```python
from build123d import *

# Parameters (mm, degrees)
PAD_DEPTH    = 4
PAD001_DEPTH = 5
POCKET_DEPTH = 4


with BuildPart() as part:
    # Sketch → Pad (new body)
    with BuildSketch(Plane.XY):
        with BuildLine():
            Line((-7, -50), (7, -50))
            Line((7, -50), (7, 0))
            Line((7, 0), (15, 0))
            ThreePointArc((15, 0), (30, 15), (15, 30))
            Line((15, 30), (-15, 30))
            ThreePointArc((-15, 30), (-30, 15), (-15, 0))
            Line((-15, 0), (-7, 0))
            Line((-7, 0), (-7, -50))
        make_face()
    extrude(amount=PAD_DEPTH)

    # Sketch001 → Pad001 (join)
    with BuildSketch(Plane.XY):
        with BuildLine():
            Line((-6, -50), (6, -50))
            Line((6, -50), (6, 1))
            Line((6, 1), (15, 1))
            ThreePointArc((15, 1), (29, 15), (15, 29))
            Line((15, 29), (-15, 29))
            ThreePointArc((-15, 29), (-29, 15), (-15, 1))
            Line((-15, 1), (-6, 1))
            Line((-6, 1), (-6, -50))
        make_face()
    extrude(amount=PAD001_DEPTH)

    # Sketch002 → Pocket (cut)
    with BuildSketch(Plane.XY.offset(5)):
        with BuildLine():
            Line((-5, -50), (5, -50))
            Line((5, -50), (5, 2))
            Line((5, 2), (15, 2))
            ThreePointArc((15, 2), (28, 15), (15, 28))
            Line((15, 28), (-15, 28))
            ThreePointArc((-15, 28), (-28, 15), (-15, 2))
            Line((-15, 2), (-5, 2))
            Line((-5, 2), (-5, -50))
        make_face()
    extrude(amount=-POCKET_DEPTH, mode=Mode.SUBTRACT)


solid = part.part
```
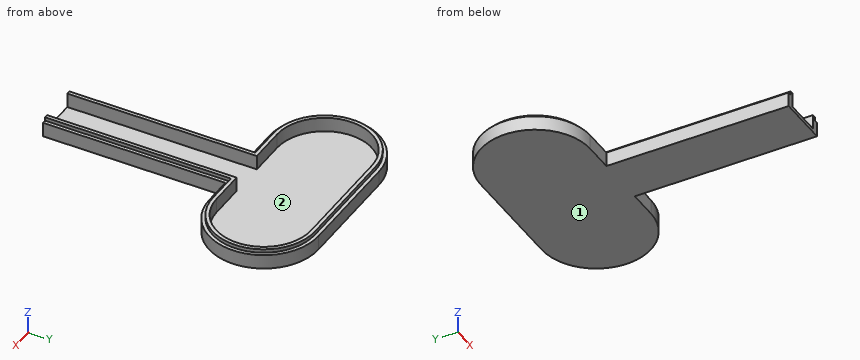
Verification items for the finished model (mm, model axes). Face numbers are marked on the shaded views. Round coordinates to 2 decimals unless told otherwise and drop trailing zeros. Write each loop counter-clockwise with the first axis right and the second up, starting at its lowest first coordinate (ties: lowest second). Pieces come first, ordered by that corner, then holes. Notation, with made-up numbers: (25.5, 46) - (53.5, 46) arc R38 cw to (53.5, 85) - close; hole circle Ø9 at (-15, -35.5). An arc over 180 degrees is marked (long way). Answer as a JSON object with one key per item and string values. Group by question number.
Q1. Section check D-D, the plane x = -9.5. Enter the section's corners in (y, z), plus the area to 3 significant figures.
Q2. Section check B-B, the plane x = 0. Enter the section's corners in (y, z), plus the area to 3 significant figures.
Q3. Section check A-A, the plane y = 15. Enter the section's corners in (x, z), plus the area to 3 significant figures.
Q4. Section check C-C, the plane z = 2. Enter the section's corners in (x, y), plus the area to 3 significant figures.
Q5. Go/stop test with flat-tipped pins: pin 1 Ø3 at (x, z) = (-2.5, 3.5) entering from -Y; pin 2 Ø0.8 at (x, z) = (11, 4.5) entering from -Y; pin 3 Ø2 at (x, y) = (-2.5, 7) entering from -Z; pin 4 Ø3 at (y, z) = (-23.5, 1) entering from -X. Record where each tip stops, or that it passes through.
Q6. Mould release check, pull along X, two halves, no side actions. Record for the marked faces 1 and 2: released by +X, released by -X, zero draft, split by the parting line, or undercut.
Q7. Thickness scan on line 1 (X direction, y = -6, z = 4.8); line 2 (Y direction, x = -12.5, z = 4.8); line 3 (Y direction, x = -11, z = 3.55). Record the ranges inside material, lowest first.
Found:
{
 "1": {"outline": "(0, 0) - (30, 0) - (30, 4) - (29, 4) - (29, 5) - (28, 5) - (28, 1) - (2, 1) - (2, 5) - (1, 5) - (1, 4) - (0, 4) - close", "area": "44.0 mm^2"},
 "2": {"outline": "(-50, 0) - (30, 0) - (30, 4) - (29, 4) - (29, 5) - (28, 5) - (28, 1) - (-50, 1) - close", "area": "87.0 mm^2"},
 "3": {"outline": "(-30, 0) - (30, 0) - (30, 4) - (29, 4) - (29, 5) - (28, 5) - (28, 1) - (-28, 1) - (-28, 5) - (-29, 5) - (-29, 4) - (-30, 4) - close", "area": "74.0 mm^2"},
 "4": {"outline": "(-15, 0) - (-7, 0) - (-7, -50) - (-5, -50) - (-5, 2) - (-15, 2) arc R13 cw to (-15, 28) - (15, 28) arc R13 cw to (15, 2) - (5, 2) - (5, -50) - (7, -50) - (7, 0) - (15, 0) arc R15 ccw to (15, 30) - (-15, 30) arc R15 ccw to start", "area": "476 mm^2"},
 "5": {"pin 1": "stops at y = 28", "pin 2": "stops at y = 1", "pin 3": "stops at z = 0", "pin 4": "stops at x = -7"},
 "6": {"face 1": "zero draft", "face 2": "undercut"},
 "7": {"line 1": "x = -6 to -5, 5 to 6", "line 2": "y = 1 to 2, 28 to 29", "line 3": "y = 0 to 2, 28 to 30"}
}
